```python
from build123d import *

# Parameters (mm, degrees)
SZKIC1_W                    = 70
SZKIC1_H                    = 58
DODANIE_WYCI_GNI_CIE1_DEPTH = 2
SZKIC2_W                    = 70
SZKIC2_H                    = 58
SZKIC2_W_2                  = 62
SZKIC2_H_2                  = 50
DODANIE_WYCI_GNI_CIE2_DEPTH = 8
SZKIC3_W                    = 70
SZKIC3_H                    = 58
SZKIC3_W_2                  = 66
SZKIC3_H_2                  = 54
DODANIE_WYCI_GNI_CIE3_DEPTH = 3


with BuildPart() as part:
    # Szkic1 → Dodanie-wyciągnięcie1 (new body)
    with BuildSketch(Plane(origin=(0, 0, 0), x_dir=(1, 0, 0), z_dir=(0, 1, 0))):
        with Locations((35, 29)):
            Rectangle(SZKIC1_W, SZKIC1_H)
    extrude(amount=DODANIE_WYCI_GNI_CIE1_DEPTH)

    # Szkic2 → Dodanie-wyciągnięcie2 (add)
    with BuildSketch(Plane(origin=(0, 2, 0), x_dir=(1, 0, 0), z_dir=(0, 1, 0))):
        with Locations((35, 29)):
            Rectangle(SZKIC2_W, SZKIC2_H)
        with Locations((35, 29)):
            Rectangle(SZKIC2_W_2, SZKIC2_H_2, mode=Mode.SUBTRACT)
    extrude(amount=DODANIE_WYCI_GNI_CIE2_DEPTH)

    # Szkic3 → Dodanie-wyciągnięcie3 (add)
    with BuildSketch(Plane(origin=(0, 10, 0), x_dir=(1, 0, 0), z_dir=(0, 1, 0))):
        with Locations((35, 29)):
            Rectangle(SZKIC3_W, SZKIC3_H)
        with Locations((35, 29)):
            Rectangle(SZKIC3_W_2, SZKIC3_H_2, mode=Mode.SUBTRACT)
    extrude(amount=DODANIE_WYCI_GNI_CIE3_DEPTH)


solid = part.part
```
Can you work these out from the model? Positions are in its coordinate system, mm. A direction names the side the tool comes from. Give positions to 0.01 mm unless a question says otherwise; leave off trailing zeros. Loops run counter-clockwise (first coordinate to the right, second up) from the corner with the lowest first, then second, coordinate; pieces in that order, holes last. Notation, with made-up numbers: M -8,6.25 L 10,6.25 A30 cw 10,42.25 Z; hole C -29,50 d3. An arc over 180 degrees is marked long. One line per item, written item: value.
(1) Suppose I cut it at C-C on x = 15. List the corners of the cut face in (y, z) for me, plus the area to 3 significant figures.
Returned:
outline: M 0,-58 L 13,-58 L 13,-56 L 10,-56 L 10,-54 L 2,-54 L 2,-4 L 10,-4 L 10,-2 L 13,-2 L 13,0 L 0,0 Z
area: 192 mm^2
(2) Which directions (+Z, -Z, +X, -X, +Y, -Y) give clear straight access to the entire face, cutting with the end or side of a thin tool? Please do faces 1 (the face through (0, 6, -29)), 2 (the face through (35, 11, -2)).
Returned:
face 1: +Z, -Z, -X, +Y, -Y
face 2: +Y
(3) Suppose I cut it at A-A on y = 11. List the corners of the cut face in (x, z) for me.
Returned:
outline: M 0,-58 L 70,-58 L 70,0 L 0,0 Z; hole M 2,-56 L 68,-56 L 68,-2 L 2,-2 Z
(4) Suppose I cut it at B-B on z = -23. List the corners of the cut face in (x, y) for me, plus the area to 3 significant figures.
Returned:
outline: M 0,0 L 70,0 L 70,13 L 68,13 L 68,10 L 66,10 L 66,2 L 4,2 L 4,10 L 2,10 L 2,13 L 0,13 Z
area: 216 mm^2
(5) Suppose I cut it at D-D on y = 6.25. List the corners of the cut face in (x, z) for me.
Returned:
outline: M 0,-58 L 70,-58 L 70,0 L 0,0 Z; hole M 4,-54 L 66,-54 L 66,-4 L 4,-4 Z
(6) I need wall thicknesses on line 1 (Z direction, x = 27, y = 11.25); line 2 (X direction, y = 12.75, z = -11); line 3 (Z direction, x = 14.5, y = 7.5). Which ranges of each line are inside material? Lowest first, please.
Returned:
line 1: -58 to -56, -2 to 0
line 2: 0 to 2, 68 to 70
line 3: -58 to -54, -4 to 0
(7) Will this pin go through, and if not, where does the flat tip stop? pin 1 (16 mm diameter, centred on x = 44, z = -34, fed in from +Y).
Returned:
pin 1: y = 2
(8) We'd pull the mould along X, two halves only. Please class faces 3 (the face through (70, 6, -29)), 4 (the face through (35, 6, -4)), 5 (the face through (35, 6, 0)), 6 (the face through (35, 2, -29)): released by +X, released by -X, zero draft, split by the parting line, or undercut.
Returned:
face 3: released by +X
face 4: undercut
face 5: zero draft
face 6: undercut
